```python
from build123d import *

# Parameters (mm, degrees)
SKETCH1_R           = 25.4
BOSS_EXTRUDE1_DEPTH = 101.6
FILLET1_R           = 3.175
FILLET2_R           = 3.175


with BuildPart() as part:
    # Sketch1 → Boss-Extrude1 (new body)
    with BuildSketch(Plane(origin=(0, 0, 0), x_dir=(1, 0, 0), z_dir=(0, 1, 0))):
        Circle(SKETCH1_R)
    extrude(amount=BOSS_EXTRUDE1_DEPTH)

    # Fillet1
    fillet1_edges = [part.edges().sort_by_distance(p)[0] for p in [
        (-25.4, 101.6, 0),
    ]]
    fillet(fillet1_edges, radius=FILLET1_R)

    # Fillet2
    fillet2_edges = [part.edges().sort_by_distance(p)[0] for p in [
        (-25.4, 0, 0),
    ]]
    fillet(fillet2_edges, radius=FILLET2_R)


solid = part.part
```
Input: part model. Units: mm. Frame: model coordinates. Give positions to 0.01 mm unless a question says otherwise; leave off trailing zeros. Loops run counter-clockwise (first coordinate to the right, second up) from the corner with the lowest first, then second, coordinate; pieces in that order, holes last. Notation, with made-up numbers: (-35.5, 6) -> (-20.5, 6) arc R18 ccw to (-20.5, 22) -> close; hole circle Ø6 at (2.5, -39.75). An arc over 180 degrees is marked (long way). Use a Markdown table: item, result.
Q1. Section query A-A, the plane y = 11. Return the cut outline in (x, z), plus the area to 3 significant figures.
Entries:
| item | result |
|---|---|
| outline | circle Ø50.8 at (0, 0) |
| area | 2,030 mm² |
Q2. Ray query, probe 1 along Z at (x, y) = (0, 5.5); probe 2 along X at (y, z) = (11.5, 18.5); probe 3 along X at (y, z) = (76.5, 9.5). Return the intervals inside material, ascending. Write a range as from..to.
Entries:
| item | result |
|---|---|
| probe 1 | z = -25.4..25.4 |
| probe 2 | x = -17.4..17.4 |
| probe 3 | x = -23.56..23.56 |
Q3. First-contact query: P1, Ø6, axis at y = 46, z = -13, coming from the +X side; P2, Ø6, axis at x = -10, y = 55.5, coming from the +Z side; P3, Ø10, axis at x = -14.5, y = 48, coming from the +Z side. Flat tips, straight axial feed; report the tip coordinate or a pass-through.
Entries:
| item | result |
|---|---|
| P1 | stops at x = 23.35 |
| P2 | stops at z = 24.42 |
| P3 | stops at z = 23.56 |
